Design review of the part built by this model. Coordinates are the model's own, in mm. A direction names the side the tool comes from. Give positions to 0.01 mm unless a question says otherwise; leave off trailing zeros. Order: outer loops, then holes, each group sorted by start corner. A loop starts at its lowest first (then second) coordinate and runs counter-clockwise, first axis right, second up. Notation, with made-up numbers: (22.5, 49) -> (68.5, 49) arc R29 cw to (68.5, 83) -> close; hole circle Ø1 at (-11, 45.25). An arc over 180 degrees is marked (long way). Return JSON: item names as keys, results as strings.
```python
from build123d import *

# Parameters (mm, degrees)
F1_DEPTH = 6.35
F3_D     = 13.49248
F4_R     = 19.05
F5_R     = 5.08


# Not quite as in the source:
# - a feature names something its author has since deleted; it is built from what else it names


with BuildPart() as f1:
    # F0 (on Front) → F1 (new body)
    with BuildSketch(Plane.XZ):
        Polygon((37.9981123171, 180.8299914), (6.2481123171, 180.8299914), (6.2481123171, 60.2186896705), (-47.5612342455, 6.2650593709), (-83.434131954, -29.7040274954), (-56.4573168042, -56.6087007767), (-20.5844190958, -20.6396139104), (0, 0), (6.2481123171, 0), (37.9981123171, 0), (37.9981123171, 33.02), align=None)
    extrude(amount=F1_DEPTH)

    # F3 (through all)
    with Locations(Plane.XZ.offset(6.35)):
        with Locations((22.2628123171, 118.2443914), (21.3484123171, 16.8009124652)):
            Hole(F3_D / 2)

    # F4
    f4_edges = [f1.edges().sort_by_distance(p)[0] for p in [
        (6.248112, -3.175, 60.21869),
        (37.998112, -3.175, 0),
        (0, -3.175, 0),
    ]]
    fillet(f4_edges, radius=F4_R)

    # F5
    f5_edges = [f1.edges().sort_by_distance(p)[0] for p in [
        (6.248112, -3.175, 180.829991),
        (37.998112, -3.175, 180.829991),
    ]]
    fillet(f5_edges, radius=F5_R)


solid = f1.part
```
Item 1: Wall thickness on L1, parallel to Z at x = 22, y = -3.25; L2, parallel to X at y = -3.75, z = 137; L3, parallel to X at y = -1.75, z = 15: over which ranges is each line inside the solid? List them lowest first. Write a range as [from, to].
Result set:
{"L1": "z = [0.25, 10.09], [23.52, 111.5], [124.99, 180.83]", "L2": "x = [6.25, 38]", "L3": "x = [-38.85, 14.85], [27.85, 37.56]"}
Item 2: Add section B-B (z = 86). Give the boundary of the cut face in (x, y).
Result set:
{"outline": "(6.25, -6.35) -> (38, -6.35) -> (38, 0) -> (6.25, 0) -> close"}
Item 3: Machinability: for faces 4 (the face through (6.248, -3, 123)), 5 (the face through (13, -3, 0)), 6 (the face through (36.55, -3.22, 179.3)), which of the approach directions +Z, -Z, +X, -X, +Y, -Y give a long, thin tool a straight path to every point of the face, cutting with its end or side? Answer none if there is none.
Result set:
{"face 4": "+Z, -X, +Y, -Y", "face 5": "-Z, +X, +Y, -Y", "face 6": "+Z, +X, +Y, -Y"}
Item 4: Add section A-A (y = -4.5). Give the boundary of the cut face in (x, z).
Result set:
{"outline": "(-83.43, -29.7) -> (-56.46, -56.61) -> (-5.58, -5.6) arc R19.05 cw to (7.91, 0) -> (18.95, 0) arc R19.05 ccw to (38, 19.05) -> (38, 175.75) arc R5.08 ccw to (32.92, 180.83) -> (11.33, 180.83) arc R5.08 ccw to (6.25, 175.75) -> (6.25, 68.09) arc R19.05 cw to (0.69, 54.64) -> close; hole circle Ø13.49 at (21.35, 16.8); hole circle Ø13.49 at (22.26, 118.24)"}
Item 5: Mouldability with a two-part tool opening along Z and no side actions: class faces 1 (the face through (7.776, -3.219, 179.381)), 2 (the face through (14.914, -3.131, 18.827)), 3 (the face through (37.998, -3, 96)) as released by +Z, released by -Z, zero draft, split by the parting line, or undercut.
Result set:
{"face 1": "released by +Z", "face 2": "undercut", "face 3": "zero draft"}
Item 6: For pin 1 (1 mm diameter, centred on x = -58, y = -1.5, fed in from +Z); pin 2 (3 mm diameter, centred on x = 15.5, y = -3, fed in from -Z); pin 3 (3 mm diameter, centred on y = -2, z = 110.5, fed in from -X); pin 4 (8 mm diameter, centred on x = 22.26, z = 118.24, fed in from -Y), all flat-tipped, find the tip position at first contact; note any pin that passes through.
Result set:
{"pin 1": "stops at z = -3.7", "pin 2": "stops at z = 0", "pin 3": "stops at x = 6.25", "pin 4": "passes through"}
Item 7: Add section C-C (x = -3). Give the boundary of the cut face in (y, z), plus the area to 3 significant figures.
Result set:
{"outline": "(-6.35, -3.43) -> (0, -3.43) -> (0, 50.95) -> (-6.35, 50.95) -> close", "area": "345 mm^2"}
